```python
from build123d import *

# Parameters (mm, degrees)
F0_R     = 19.5
F0_R_2   = 18.7
F1_DEPTH = 38
F0_R_3   = 22.5
F2_DEPTH = 1
F3_R     = 0.4


with BuildPart() as f1:
    # F0 (on Top) → F1 (new body)
    with BuildSketch(Plane.XY):
        Circle(F0_R)
        Circle(F0_R_2, mode=Mode.SUBTRACT)
    extrude(amount=-F1_DEPTH)

    # F0 (on Top) → F2 (join)
    with BuildSketch(Plane.XY):
        Circle(F0_R_3)
        Circle(F0_R, mode=Mode.SUBTRACT)
        Circle(F0_R)
        Circle(F0_R_2, mode=Mode.SUBTRACT)
    extrude(amount=F2_DEPTH)

    # F3
    f3_edges = [f1.edges().sort_by_distance(p)[0] for p in [
        (-22.5, 0, 1),
    ]]
    fillet(f3_edges, radius=F3_R)


solid = f1.part
```
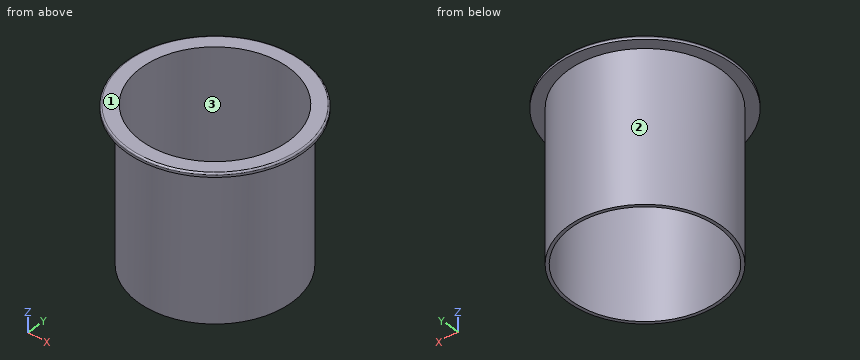
CAD build for the part. Positions are in the model's coordinates, mm. Face numbers are marked on the shaded views. Coordinates: 2 decimals unless noted, no trailing zeros. Loops run counter-clockwise (first coordinate to the right, second up) from the corner with the lowest first, then second, coordinate; pieces in that order, holes last. Notation, with made-up numbers: (-5.75, -24.75) - (11.25, -24.75) arc R27 ccw to (11.25, 10.25) - close; hole circle Ø8 at (49, 13.25). An arc over 180 degrees is marked (long way). Return JSON: item names as keys, results as strings.
1. Band-saw the part on A-A (y = 0). Give the cut face in (x, z), and give its area (3 significant figures).
Result:
{"outline": "(-22.5, 0) - (-19.5, 0) - (-19.5, -38) - (-18.7, -38) - (-18.7, 1) - (-22.1, 1) arc R0.4 ccw to (-22.5, 0.6) - close; (18.7, -38) - (19.5, -38) - (19.5, 0) - (22.5, 0) - (22.5, 0.6) arc R0.4 ccw to (22.1, 1) - (18.7, 1) - close", "area": "68.3 mm2"}
2. Band-saw the part on C-C (z = -33.5). Give the cut face in (x, y), and give its area (3 significant figures).
Result:
{"outline": "circle Ø39 at (0, 0); hole circle Ø37.4 at (0, 0)", "area": "96.0 mm2"}
3. Mould opens along X. For the marked faces 1, 2 and 3 say: released by +X, released by -X, zero draft, split by the parting line, or undercut.
Result:
{"face 1": "zero draft", "face 2": "split by the parting line", "face 3": "undercut"}
4. Drop flat-ended pins along their axis: pin 1 (3 mm diameter, centred on y = -16, z = -27, fed in from +X); pin 2 (6 mm diameter, centred on y = -1, z = -5.5, fed in from -X); pin 3 (1.5 mm diameter, centred on y = 15.5, z = -10.5, fed in from +X); pin 4 (2 mm diameter, centred on x = -14.5, y = 9.5, fed in from +Z). Give the stop position or say it passes through.
Result:
{"pin 1": "stops at x = 13.04", "pin 2": "stops at x = -19.5", "pin 3": "stops at x = 12.75", "pin 4": "passes through"}
5. Probe L1, parallel to X at y = 15, z = -4; L2, parallel to X at y = -1.5, z = -8; L3, parallel to Y at x = 0, z = -17. List the from-to ranges inside material, lowest first. Write a range as from..to.
Result:
{"L1": "x = -12.46..-11.17, 11.17..12.46", "L2": "x = -19.44..-18.64, 18.64..19.44", "L3": "y = -19.5..-18.7, 18.7..19.5"}
